Could you check a few things on this model? Use its own coordinates, in mm. A direction names the side the tool comes from. Coordinates: 2 decimals unless noted, no trailing zeros. Loops run counter-clockwise (first coordinate to the right, second up) from the corner with the lowest first, then second, coordinate; pieces in that order, holes last. Notation, with made-up numbers: M -13.5,5.5 L 21.5,5.5 A11 cw 21.5,25.5 Z; hole C -33,39 d4. An arc over 180 degrees is marked long. Write each question's results on one line, items separated by ' | '.
Autodesk Inventor part; units mm, degrees
ref_plane "Work Plane1" through (50, 0, 0) normal (1, 0, 0) x (0, 1, 0)
ref_plane "XZ Plane" through (0, 0, 0) normal (0, 1, 0) x (-1, 0, 0)
ref_plane "XY Plane" through (0, 0, 0) normal (0, 0, 1) x (1, 0, 0)
sketch "Sketch1" plane through (0, 0, 0) normal (0, 0, 1) x (1, 0, 0)
  circle A0 centre (0, 0) radius 50
  dimension "d0" = 100
extrude "Extrusion1" add sketch "Sketch1" along normal blind 300
sketch "Sketch2" plane through (0, 0, 300) normal (0, 0, 1) x (1, 0, 0)
  circle A0 centre (0, 0) radius 50
  circle A1 centre (0, 0) radius 46
  dimension "d3" = 92
extrude "Extrusion2" cut sketch "Sketch2" against normal blind 296 contours A1
sketch "Sketch3" plane through (0, 0, 300) normal (0, 0, 1) x (1, 0, 0)
  circle A0 centre (0, 0) radius 46
extrude "Extrusion3" add sketch "Sketch3" against normal blind 4
sketch "Sketch4" plane through (0, 0, 300) normal (0, 0, 1) x (1, 0, 0)
  circle A0 centre (0, 0) radius 25
  dimension "d8" = 50
extrude "Extrusion4" add sketch "Sketch4" along normal blind 50
sketch "Sketch5" plane through (0, 0, 350) normal (0, 0, 1) x (1, 0, 0)
  circle A0 centre (0, 0) radius 12.5
  dimension "d11" = 25
extrude "Extrusion5" cut sketch "Sketch5" against normal blind 100
sketch "Sketch6" plane through (0, 0, 350) normal (0, 0, 1) x (1, 0, 0)
  circle A0 centre (0, 0) radius 50
extrude "Extrusion6" add sketch "Sketch6" along normal blind 10
sketch "Sketch7" plane through (0, 0, 360) normal (0, 0, 1) x (1, 0, 0)
  circle A0 centre (0, 0) radius 12.5
  circle A1 centre (0, 0) radius 12.5
extrude "Extrusion7" cut sketch "Sketch7" against normal blind 300
sketch "Sketch8" plane through (0, 0, 360) normal (0, 0, 1) x (1, 0, 0)
  line L0 (0, 0) -> (0, -36)
  line L1 (0, 0) -> (0, 36)
  line L2 (0, 0) -> (36, 0)
  line L3 (0, 0) -> (-36, 0)
  circle A0 centre (0, 0) radius 12.5
  line L4 (0, 0) -> (0, 36)
  circle A1 centre (0, 36) radius 4
  dimension "d31" = 8
ref_plane "Work Plane1" through (50, 0, 0) normal (1, 0, 0) x (0, 1, 0)
extrude "Extrusion9" cut sketch "Sketch8" along normal mid plane 25 contours A1
sketch "Sketch11" plane through (0, 0, 360) normal (0, 0, 1) x (1, 0, 0)
  point P0 (0, 0)
pattern_circular "Circular Pattern1" count 6 over 360 about axis through (0, 0, 350) along (0, 0, -1) of "Extrusion9"
sketch "Sketch12" plane through (50, 0, 0) normal (1, 0, 0) x (0, 1, 0)
  line L0 (0, 0) -> (0, 50)
  circle A0 centre (0, 50) radius 5.5
  dimension "d37" = 50
  dimension "d39" = 11
extrude "Extrusion10" cut sketch "Sketch12" against normal blind 50
properties part number "again"
(1) Imagine slicing it at D-D, the plane z = 147. List the corners of the cut face in (x, y) for me.
Reported:
outline: C 0,0 d100; hole C 0,0 d92
(2) Imagine slicing it at C-C, the plane y = -18. List the corners of the cut face in (x, z) for me.
Reported:
outline: M -46.65,0 L 46.65,0 L 46.65,300 L 17.35,300 L 17.35,350 L 27.18,350 L 27.18,360 L -27.18,360 L -27.18,350 L -17.35,350 L -17.35,300 L -46.65,300 Z; M -46.65,350 L -35.18,350 L -35.18,360 L -46.65,360 Z; M 35.18,350 L 46.65,350 L 46.65,360 L 35.18,360 Z; hole M -42.33,4 L 42.33,4 L 42.33,296 L -42.33,296 Z
(3) Imagine slicing it at B-B, the plane x = 0. List the corners of the cut face in (y, z) for me.
Reported:
outline: M -50,0 L 50,0 L 50,300 L 25,300 L 25,350 L 32,350 L 32,360 L 12.5,360 L 12.5,296 L 46,296 L 46,4 L -46,4 L -46,296 L -12.5,296 L -12.5,360 L -32,360 L -32,350 L -25,350 L -25,300 L -50,300 Z; M -50,350 L -40,350 L -40,360 L -50,360 Z; M 40,350 L 50,350 L 50,360 L 40,360 Z
(4) Imagine slicing it at A-A, the plane y = 0. List the corners of the cut face in (x, z) for me, and give its area (3 significant figures).
Reported:
outline: M -50,0 L 50,0 L 50,44.5 L 46,44.5 L 46,4 L -46,4 L -46,296 L -12.5,296 L -12.5,360 L -50,360 L -50,350 L -25,350 L -25,300 L -50,300 Z; M 12.5,296 L 46,296 L 46,55.5 L 50,55.5 L 50,300 L 25,300 L 25,350 L 50,350 L 50,360 L 12.5,360 Z | area: 4,990 mm2
(5) Which directions (+Z, -Z, +X, -X, +Y, -Y) give clear straight access to the entire face, cutting with the end or side of a thin tool? Please do faces 1 (the cylindrical face through (28, -15.57, 354.93)), 2 (the flat face through (-22.9, -10.4, 300)), 3 (the cylindrical face through (47.865, -5.495, 50.242)), 4 (the flat face through (-1, 1, 0)).
Reported:
face 1: +Z | face 2: none | face 3: +X | face 4: -Z, +X, -X, +Y, -Y
(6) Please list where these lines run through material, in increasing order: probe 1 along Z at (x, y) = (-17.5, -34); probe 2 along Z at (x, y) = (47, 0); probe 3 along Y at (x, z) = (0, 352). Write a range as from..to.
Reported:
probe 1: z = 0..4, 296..300, 350..360 | probe 2: z = 0..44.5, 55.5..300, 350..360 | probe 3: y = -50..-40, -32..-12.5, 12.5..32, 40..50
(7) Will these pins go through, and if not, where does the flat tip stop? P1, Ø13, axis at x = -31.18, y = 18, coming from the -Z side; P2, Ø5, axis at x = 0, y = 36, coming from the +Z side; P3, Ø2, axis at x = -18.5, z = 308, coming from the -Y side; P4, Ø9, axis at y = 0, z = 50, coming from the +X side.
Reported:
P1: stops at z = 0 | P2: stops at z = 300 | P3: stops at y = -17.85 | P4: stops at x = -45.78
(8) If we mould it in two halves opening along Y, with no side actions, what happens to faces 5 (the flat face through (10, -10, 360)), 6 (the flat face through (10, -10, 296)), 7 (the cylindrical face through (47.69, -15.02, 354.93))? For each: released by +Y, released by -Y, zero draft, split by the parting line, or undercut.
Reported:
face 5: zero draft | face 6: undercut | face 7: split by the parting line
